Read the model definition and answer for the solid it produces. Units are mm, in the model's axes. A direction names the side the tool comes from. Round coordinates to 2 decimals unless told otherwise and drop trailing zeros. Write each loop counter-clockwise with the first axis right and the second up, starting at its lowest first coordinate (ties: lowest second). Pieces come first, ordered by that corner, then holes. Notation, with made-up numbers: (49.25, -5.75) -> (69.25, -5.75) arc R24 cw to (69.25, 30.25) -> close; hole circle Ø8 at (1.25, 32.25). An arc over 180 degrees is marked (long way). Return JSON: item names as keys, results as strings.
from build123d import *

# Parameters (mm, degrees)
PAD_DEPTH = 20
FILLET_R  = 1


with BuildPart() as part:
    # Sketch → Pad (new body)
    with BuildSketch(Plane.XY):
        Polygon((0, 0), (0, 33.02), (10, 33.02), (10, 28.02), (5, 28.02), (5, 25), (10, 25), (10, 18.02), (5, 18.02), (5, 15), (10, 15), (10, 10), (5, 10), (5, 0), align=None)
    extrude(amount=PAD_DEPTH)

    # Fillet
    fillet_edges = [part.edges().sort_by_distance(p)[0] for p in [
        (0, 33.02, 10),
        (10, 33.02, 10),
        (5, 33.02, 0),
        (5, 33.02, 20),
        (0, 0, 10),
        (0, 16.51, 0),
        (0, 16.51, 20),
        (2.5, 0, 0),
        (2.5, 0, 20),
    ]]
    fillet(fillet_edges, radius=FILLET_R)


solid = part.part
Item 1: Section D-D (x = 0.5) is taken. Give the vertices of the cut face in (y, z).
Worked answers:
{"outline": "(0.13, 1) arc R0.87 ccw to (1, 0.13) -> (32.02, 0.13) arc R0.87 ccw to (32.89, 1) -> (32.89, 19) arc R0.87 ccw to (32.02, 19.87) -> (1, 19.87) arc R0.87 ccw to (0.13, 19) -> close"}
Item 2: Section B-B (z = 12.25) is taken. Give the vertices of the cut face in (x, y), then the cut area to 3 significant figures.
Worked answers:
{"outline": "(0, 1) arc R1 ccw to (1, 0) -> (5, 0) -> (5, 10) -> (10, 10) -> (10, 15) -> (5, 15) -> (5, 18.02) -> (10, 18.02) -> (10, 25) -> (5, 25) -> (5, 28.02) -> (10, 28.02) -> (10, 32.02) arc R1 ccw to (9, 33.02) -> (1, 33.02) arc R1 ccw to (0, 32.02) -> close", "area": "249 mm2"}
Item 3: Section A-A (x = 8.5) is taken. Give the vertices of the cut face in (y, z), then the cut area to 3 significant figures.
Worked answers:
{"outline": "(10, 0) -> (15, 0) -> (15, 20) -> (10, 20) -> close; (18.02, 0) -> (25, 0) -> (25, 20) -> (18.02, 20) -> close; (28.02, 0) -> (32.02, 0) arc R1 ccw to (33.02, 1) -> (33.02, 19) arc R1 ccw to (32.02, 20) -> (28.02, 20) -> close", "area": "339 mm2"}
Item 4: Flat-ended cylindrical pins translate along their axes: pin 1 (1.5 mm diameter, centred on x = 8, z = 10, fed in from -Y); pin 2 (5 mm diameter, centred on y = 7, z = 14.5, fed in from +X). Find the tip coordinate at first contact, or state that the pin passes through.
Worked answers:
{"pin 1": "stops at y = 10", "pin 2": "stops at x = 5"}
Item 5: Straight lines are drawn through the part: L1, parallel to Y at x = 7.5, z = 8.75; L2, parallel to X at y = 8, z = 8; L3, parallel to Z at x = 0.75, y = 24. For each, find the intervals that lie inside material, in ascending order. Write a range as [from, to].
Worked answers:
{"L1": "y = [10, 15], [18.02, 25], [28.02, 33.02]", "L2": "x = [0, 5]", "L3": "z = [0.03, 19.97]"}
Item 6: For a pull along Y with two mould halves and no side action, classify faces 1 (the flat face through (8, 18.02, 10)), 2 (the cylindrical face through (5.563, 32.735, 0.301)), 3 (the flat face through (10, 13, 10)) as released by +Y, released by -Y, zero draft, split by the parting line, or undercut.
Worked answers:
{"face 1": "undercut", "face 2": "released by +Y", "face 3": "zero draft"}
Item 7: Section C-C (y = 3) is taken. Give the vertices of the cut face in (x, z), then the cut area to 3 significant figures.
Worked answers:
{"outline": "(0, 1) arc R1 ccw to (1, 0) -> (5, 0) -> (5, 20) -> (1, 20) arc R1 ccw to (0, 19) -> close", "area": "99.6 mm2"}
Item 8: A tool of negligible diameter and unlimited length cuts with its end or side. For faces 4 (the cylindrical face through (0.285, 0.301, 10.126)), 5 (the flat face through (8, 10, 10)), 6 (the flat face through (5, 27, 10)), from which of +Z, -Z, +X, -X, +Y, -Y can it reach the whole face along a straight path? Write none if from no direction.
Worked answers:
{"face 4": "+Z, -Z, -X, -Y", "face 5": "+Z, -Z, +X, -Y", "face 6": "+Z, -Z, +X"}
